from build123d import *

# Parameters (mm, degrees)
SKETCH1_R      = 3.175
EXTRUDE1_DEPTH = 38.1
CHAMFER1_SIZE  = 0.635
EXTRUDE7_DEPTH = 26.4


with BuildPart() as part:
    # Sketch1 → Extrude1 (new body, symmetric)
    with BuildSketch(Plane.XY):
        Circle(SKETCH1_R)
    extrude(amount=EXTRUDE1_DEPTH, both=True)

    # Chamfer1
    chamfer1_edges = [part.edges().sort_by_distance(p)[0] for p in [
        (-3.175, 0, -38.1),
        (-3.175, 0, 38.1),
    ]]
    chamfer(chamfer1_edges, length=CHAMFER1_SIZE)

    # Sketch13 → Extrude7 (cut, through all)
    with BuildSketch(Plane.XY.offset(12.7)):
        with BuildLine():
            Line((-1.5875, 2.749630657), (1.5875, 2.749630657))
            ThreePointArc((1.5875, 2.749630657), (0, 3.175), (-1.5875, 2.749630657))
        make_face()
    extrude(amount=EXTRUDE7_DEPTH, mode=Mode.SUBTRACT)


solid = part.part
Work out the finished part from the listing and answer in its coordinate system (mm). A direction names the side the tool comes from. Round coordinates to 2 decimals unless told otherwise and drop trailing zeros. Write each loop counter-clockwise with the first axis right and the second up, starting at its lowest first coordinate (ties: lowest second). Pieces come first, ordered by that corner, then holes. Notation, with made-up numbers: (-9, -30) -> (13, -30) arc R5 cw to (13, -23) -> close; hole circle Ø5 at (61, 17). An arc over 180 degrees is marked (long way). Answer as CSV lines item,"result". Start each with the question number.
(1) A tool of negligible diameter and unlimited length cuts with its end or side. For faces 1 (the flat face through (0, 2.75, 25)), 2 (the flat face through (0, 0, -38.1)), from which of +Z, -Z, +X, -X, +Y, -Y can it reach the whole face along a straight path? Write none if from no direction.
(2) The part is cut by section B-B, the plane z = -30.5. Give the vertices of the cut face in (x, y) (3 decimals), then the cut area to 3 significant figures.
(3) The part is cut by section A-A, the plane x = 0. Give the vertices of the cut face in (y, z) (3 decimals).
(4) Find the intervals of material crossed by probe 1 along Y at (x, z) = (2.75, 15); probe 2 along X at (y, z) = (2.5, 32), in increasing order.
(5) Each of these flat-tipped pins is pushed along its axis until it touches: pin 1 (1 mm diameter, centred on x = 2, z = -21, fed in from +Y); pin 2 (2.5 mm diameter, centred on x = -0.5, z = 26.5, fed in from +Y); pin 3 (2 mm diameter, centred on y = -2.5, z = -27, fed in from -X). Where does it stop, or does it pass through?
Output values:
1,face 1,"+Z, +X, -X, +Y"
1,face 2,"-Z, +X, -X, +Y, -Y"
2,outline,"circle Ø6.35 at (0, 0)"
2,area,"31.7 mm²"
3,outline,"(-3.175, -37.465) -> (-2.54, -38.1) -> (2.54, -38.1) -> (3.175, -37.465) -> (3.175, 12.7) -> (2.75, 12.7) -> (2.75, 37.89) -> (2.54, 38.1) -> (-2.54, 38.1) -> (-3.175, 37.465) -> close"
4,probe 1,"y = -1.59 to 1.59"
4,probe 2,"x = -1.96 to 1.96"
5,pin 1,"stops at y = 2.8"
5,pin 2,"stops at y = 2.75"
5,pin 3,"stops at x = -2.8"
